CAD build for the part. Positions are in the model's coordinates, mm. A direction names the side the tool comes from. Round coordinates to 2 decimals unless told otherwise and drop trailing zeros. Order: outer loops, then holes, each group sorted by start corner. A loop starts at its lowest first (then second) coordinate and runs counter-clockwise, first axis right, second up. Notation, with made-up numbers: (40.5, -20.5) - (67.5, -20.5) arc R8 ccw to (67.5, -14.5) - close; hole circle Ø8 at (1.5, 18.5). An arc over 180 degrees is marked (long way). Use one line per item in the form item = value. Start each with the question number.
from build123d import *

# Parameters (mm, degrees)
F6_DEPTH = 450
F1_R     = 2.5
F2_R     = 1.5
F3_R     = 1.5
F7_R     = 2.5


with BuildPart() as f6:
    # F0 (on Right) → F6 (new body)
    with BuildSketch(Plane.YZ):
        Polygon((1.5, 0), (0, 0), (0, -60), (500, -60), (500, 0), (498.5, 0), (498.5, -58.5), (1.5, -58.5), align=None)
    extrude(amount=F6_DEPTH)

    # F1
    f1_edges = [f6.edges().sort_by_distance(p)[0] for p in [
        (225, 500, -60),
    ]]
    fillet(f1_edges, radius=F1_R)

    # F2
    f2_edges = [f6.edges().sort_by_distance(p)[0] for p in [
        (225, 498.5, -58.5),
    ]]
    fillet(f2_edges, radius=F2_R)

    # F3
    f3_edges = [f6.edges().sort_by_distance(p)[0] for p in [
        (225, 1.5, -58.5),
    ]]
    fillet(f3_edges, radius=F3_R)

    # F7
    f7_edges = [f6.edges().sort_by_distance(p)[0] for p in [
        (225, 0, -60),
    ]]
    fillet(f7_edges, radius=F7_R)


solid = f6.part
(1) Flat gauge pin, fed straight in: P1, Ø4, axis at x = 194.5, y = 113, coming from the +Z side. Where does the tip first touch, or does it go through?
(2) Slice it at C-C (y = 96). Give the cut face in (x, z).
(3) Wall check: line 1 (Y direction, x = 339.5, z = -53); line 2 (Z direction, x = 47, y = 138). Give the ranges that are in metal, low to high. Write a range as [from, to].
(4) Which spindle directions (+Z, -Z, +X, -X, +Y, -Y) get a long thin tool onto all of the face, cutting with end or side? Do faces 5 (the flat face through (0, 249, -59)), 6 (the flat face through (222, 253, -58.5)). Say none if no direction does.
(5) Mould opens along Y. For faces 1 (the flat face through (222, 1.5, -29)), 2 (the flat face through (222, 500, -29)), 3 (the flat face through (222, 0, -28)), 4 (the flat face through (450, 249, -59)) say: pulls with the +Y half, pulls with the -Y half, needs draft (parallel to the pull), parting line crosses it, or undercut.
(6) Slice it at A-A (z = -17). Give the cut face in (x, y), and give its area (3 significant figures).
(7) Slice it at B-B (x = 101.5). Give the cut face in (y, z), and give its area (3 significant figures).
Results list:
q1.P1 = -58.5
q2.outline = (0, -60) - (450, -60) - (450, -58.5) - (0, -58.5) - close
q3.line_1 = [0, 1.5], [498.5, 500]
q3.line_2 = [-60, -58.5]
q4.face_5 = +Z, -Z, -X, +Y, -Y
q4.face_6 = +Z, +X, -X
q5.face_1 = undercut
q5.face_2 = pulls with the +Y half
q5.face_3 = pulls with the -Y half
q5.face_4 = needs draft
q6.outline = (0, 0) - (450, 0) - (450, 1.5) - (0, 1.5) - close; (0, 498.5) - (450, 498.5) - (450, 500) - (0, 500) - close
q6.area = 1,350 mm²
q7.outline = (0, -57.5) arc R2.5 ccw to (2.5, -60) - (497.5, -60) arc R2.5 ccw to (500, -57.5) - (500, 0) - (498.5, 0) - (498.5, -57) arc R1.5 cw to (497, -58.5) - (3, -58.5) arc R1.5 cw to (1.5, -57) - (1.5, 0) - (0, 0) - close
q7.area = 924 mm²
